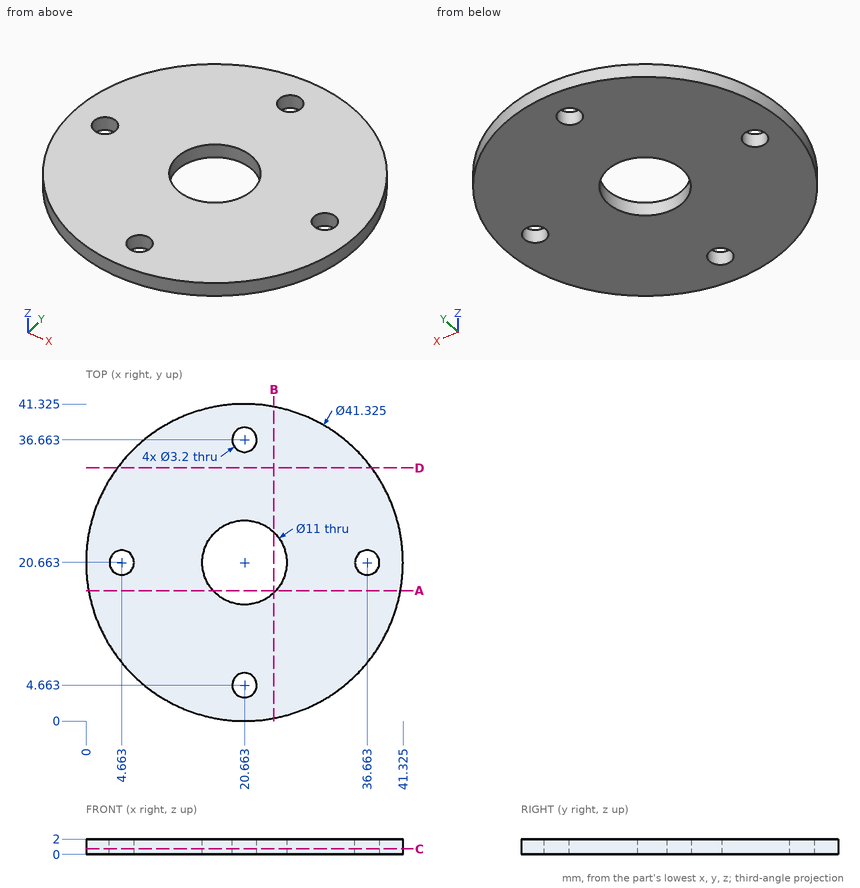
Geometry: see drawing. Coordinates: mm, zero at the bounding-box minimum. Give positions to 0.01 mm unless a question says otherwise; leave off trailing zeros. Write each loop counter-clockwise with the first axis right and the second up, starting at its lowest first coordinate (ties: lowest second). Pieces come first, ordered by that corner, then holes. Notation, with made-up numbers: M -39,-39 L -26,-39 A13 ccw -26,-33 Z; hole C 40.5,-37.75 d3. An arc over 180 degrees is marked long. Answer in a Markdown table with one row per item. Add a question column.
(1) Ray query, line 1 (Y direction, x = 19.5, z = 1.4) (1 decimal); line 2 (X direction, y = 19, z = 0.25) (1 decimal). Return the intervals inside material, ascending.
(2) Section A-A on y = 17. Return loops of the section in (x, z) (1 decimal).
(3) Section C-C on z = 0.7. Return loops of the section in (x, y) (1 decimal), and give its area (3 significant figures).
(4) First-contact query: pin 1 (1 mm diameter, centred on y = 28.5, z = 1.5, fed in from -X). Flat tip, straight axial feed; report the tip coordinate or a pass-through.
(5) Section D-D on y = 33. Return loops of the section in (x, z).
(6) Section B-B on x = 24.5. Return loops of the section in (y, z) (1 decimal).
Result set:
| question | item | result |
|---|---|---|
| 1 | line 1 | y = 0 to 3.6, 5.8 to 15.3, 26 to 35.6, 37.8 to 41.3 |
| 1 | line 2 | x = 0.1 to 15.4, 25.9 to 41.3 |
| 2 | outline | M 0.3,0 L 16.6,0 L 16.6,2 L 0.3,2 Z; M 24.8,0 L 41,0 L 41,2 L 24.8,2 Z |
| 3 | outline | C 20.7,20.7 d41.3; hole C 4.7,20.7 d3.2; hole C 20.7,20.7 d11; hole C 20.7,4.7 d3.2; hole C 20.7,36.7 d3.2; hole C 36.7,20.7 d3.2 |
| 3 | area | 1,210 mm^2 |
| 4 | pin 1 | stops at x = 1.35 |
| 5 | outline | M 4.09,0 L 37.24,0 L 37.24,2 L 4.09,2 Z |
| 6 | outline | M 0.4,0 L 16.7,0 L 16.7,2 L 0.4,2 Z; M 24.6,0 L 41,0 L 41,2 L 24.6,2 Z |
